The drawing under review shows one solid part. Ordinate dimensions are in mm from its lowest x, y, z. Round coordinates to 2 decimals unless told otherwise and drop trailing zeros. Order: outer loops, then holes, each group sorted by start corner. A loop starts at its lowest first (then second) coordinate and runs counter-clockwise, first axis right, second up. Notation, with made-up numbers: M 76,57.5 L 115,57.5 A13 cw 115,72.5 Z; hole C 57,-24 d3. An arc over 180 degrees is marked long. Write item = value, one per line. Start each with the question number.
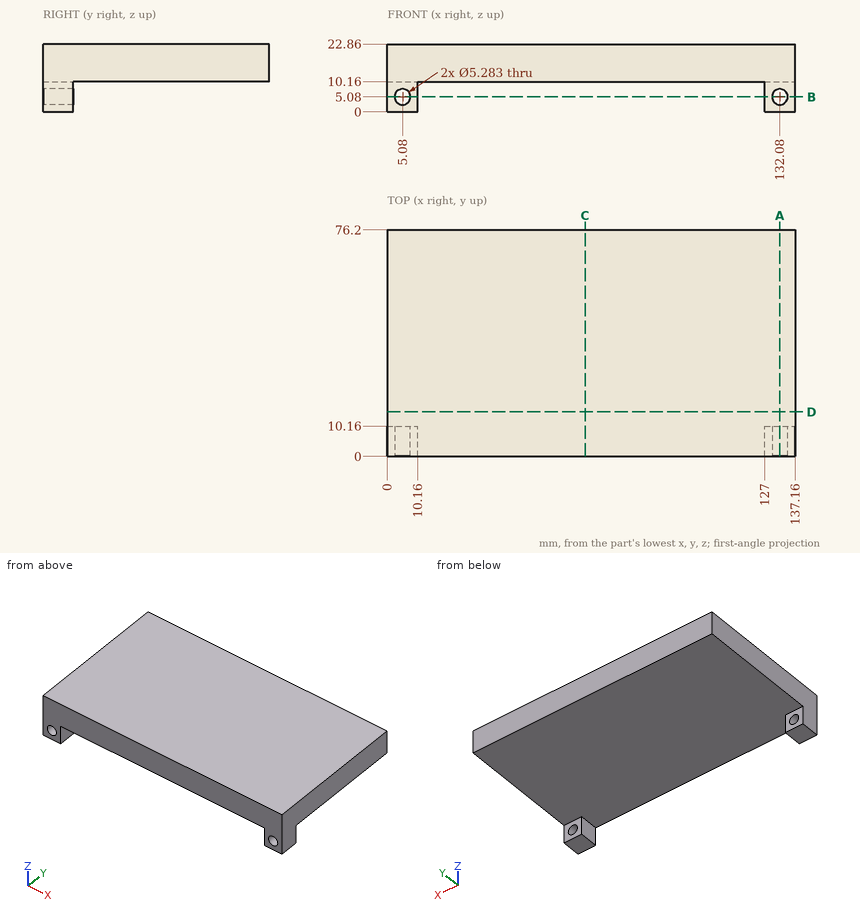
(1) Consider section D-D, the plane y = 15. Write out the cut boundary in (x, z), then the cut area to 3 significant figures.
(2) For line 1 along Z through (x, y) = (132, 4); line 2 along Y through (x, z) = (6, 10); line 3 along Z through (x, y) = (56, 45), list the stretches that pass through material, from the lowest coordinate up. Write a range as [from, to].
(3) Consider section C-C, the plane x = 66.5. Write out the cut boundary in (y, z).
(4) Insertion check: pin 1 (5 mm diameter, centred on x = 130.5, z = 6.5, fed in from +Y); pin 2 (6 mm diameter, centred on x = 82.5, z = 6.5, fed in from +Y). Each pin has a flat end and moves straight along its axis. Give the tip position at first contact, or say it passes through.
(5) Consider section B-B, the plane z = 5.08. Write out the cut boundary in (x, y), then the cut area to 3 significant figures.
(6) Consider section A-A, the plane x = 132.08. Write out the cut boundary in (y, z), then the cut area to 3 significant figures.
Completed:
q1.outline = M 0,10.16 L 137.16,10.16 L 137.16,22.86 L 0,22.86 Z
q1.area = 1,740 mm2
q2.line_1 = [0, 2.44], [7.72, 22.86]
q2.line_2 = [0, 10.16]
q2.line_3 = [10.16, 22.86]
q3.outline = M 0,10.16 L 76.2,10.16 L 76.2,22.86 L 0,22.86 Z
q4.pin_1 = 10.16
q4.pin_2 = through
q5.outline = M 0,0 L 2.44,0 L 2.44,10.16 L 0,10.16 Z; M 7.72,0 L 10.16,0 L 10.16,10.16 L 7.72,10.16 Z; M 127,0 L 129.44,0 L 129.44,10.16 L 127,10.16 Z; M 134.72,0 L 137.16,0 L 137.16,10.16 L 134.72,10.16 Z
q5.area = 99.1 mm2
q6.outline = M 0,0 L 10.16,0 L 10.16,2.44 L 0,2.44 Z; M 0,7.72 L 10.16,7.72 L 10.16,10.16 L 76.2,10.16 L 76.2,22.86 L 0,22.86 Z
q6.area = 1,020 mm2
